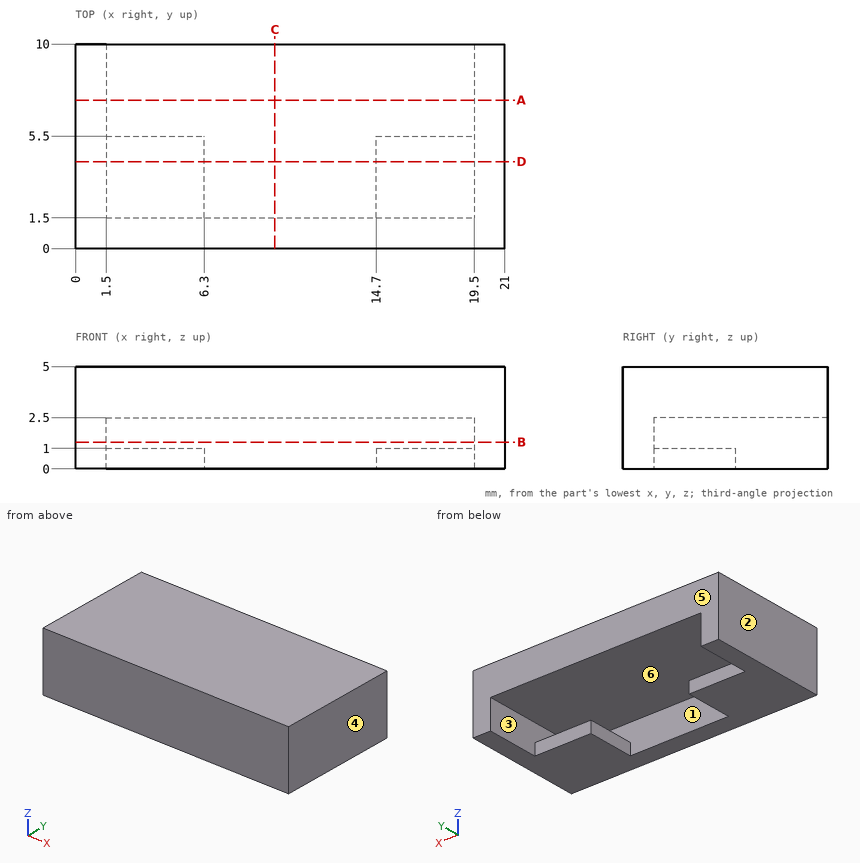
Study the drawing (mm; zero at the part's minimum x, y, z) and answer. A direction names the side the tool comes from. Coordinates: 2 decimals unless noted, no trailing zeros. Order: outer loops, then holes, each group sorted by start corner. A loop starts at its lowest first (then second) coordinate and runs counter-clockwise, first axis right, second up. Notation, with made-up numbers: (-37, 1.5) -> (-16, 1.5) arc R12 cw to (-16, 14.5) -> close; hole circle Ø1 at (77, 5). An arc over 180 degrees is marked (long way). Answer in a Markdown table with one row per item. Add a question column.
Item 1: Find section B-B (z = 1.3). Write down the section's boundary in (x, y).
Item 2: Find section A-A (y = 7.25). Write down the section's boundary in (x, z), then the cut area to 3 significant figures.
Item 3: Find section D-D (y = 4.25). Write down the section's boundary in (x, z), then the cut area to 3 significant figures.
Item 4: Find the intervals of material crossed by L1, parallel to Z at x = 16.5, y = 3.5; L2, parallel to X at y = 7.75, z = 2; L3, parallel to Y at x = 7.25, z = 1.2, in increasing order. Write a range as from..to.
Item 5: Each of these flat-tipped pins is pushed along its axis until it touches: P1, Ø5, axis at x = 12.5, y = 7, coming from the -Z side; P2, Ø0.5, axis at x = 17, z = 0.5, coming from the +Y side. Where does it stop, or does it pass through?
Item 6: Determine the mould class of the marked faces 1, 2, 3 and 4 for opening direction X: +X half, -X half, draft (parallel to the pull), parting line (faces both ways), or undercut.
Item 7: Which of the six approach directions +Z, -Z, +X, -X, +Y, -Y give full straight-line access (tool end or side, diameter ignored) to the marked faces 5 and 6?
Item 8: Find section C-C (x = 9.75). Write down the section's boundary in (y, z).
Result set:
| question | item | result |
|---|---|---|
| 1 | outline | (0, 0) -> (21, 0) -> (21, 10) -> (19.5, 10) -> (19.5, 1.5) -> (1.5, 1.5) -> (1.5, 10) -> (0, 10) -> close |
| 2 | outline | (0, 0) -> (1.5, 0) -> (1.5, 2.5) -> (19.5, 2.5) -> (19.5, 0) -> (21, 0) -> (21, 5) -> (0, 5) -> close |
| 2 | area | 60.0 mm² |
| 3 | outline | (0, 0) -> (6.3, 0) -> (6.3, 1) -> (1.5, 1) -> (1.5, 2.5) -> (19.5, 2.5) -> (19.5, 1) -> (14.7, 1) -> (14.7, 0) -> (21, 0) -> (21, 5) -> (0, 5) -> close |
| 3 | area | 69.6 mm² |
| 4 | L1 | z = 0..1, 2.5..5 |
| 4 | L2 | x = 0..1.5, 19.5..21 |
| 4 | L3 | y = 0..1.5 |
| 5 | P1 | stops at z = 2.5 |
| 5 | P2 | stops at y = 5.5 |
| 6 | face 1 | undercut |
| 6 | face 2 | -X half |
| 6 | face 3 | undercut |
| 6 | face 4 | +X half |
| 7 | face 5 | +Z, -Z, +X, -X, +Y |
| 7 | face 6 | +Y |
| 8 | outline | (0, 0) -> (1.5, 0) -> (1.5, 2.5) -> (10, 2.5) -> (10, 5) -> (0, 5) -> close |
